The drawing under review shows one solid part. Ordinate dimensions are in mm from its lowest x, y, z. Give positions to 0.01 mm unless a question says otherwise; leave off trailing zeros. Write each loop counter-clockwise with the first axis right and the second up, starting at its lowest first coordinate (ties: lowest second). Pieces come first, ordered by that corner, then holes. Notation, with made-up numbers: (31.25, -2) -> (37.25, -2) arc R15 cw to (37.25, 11) -> close; hole circle Ø9 at (27, 40.5). An arc over 180 degrees is marked (long way). Write item = value, one per line.
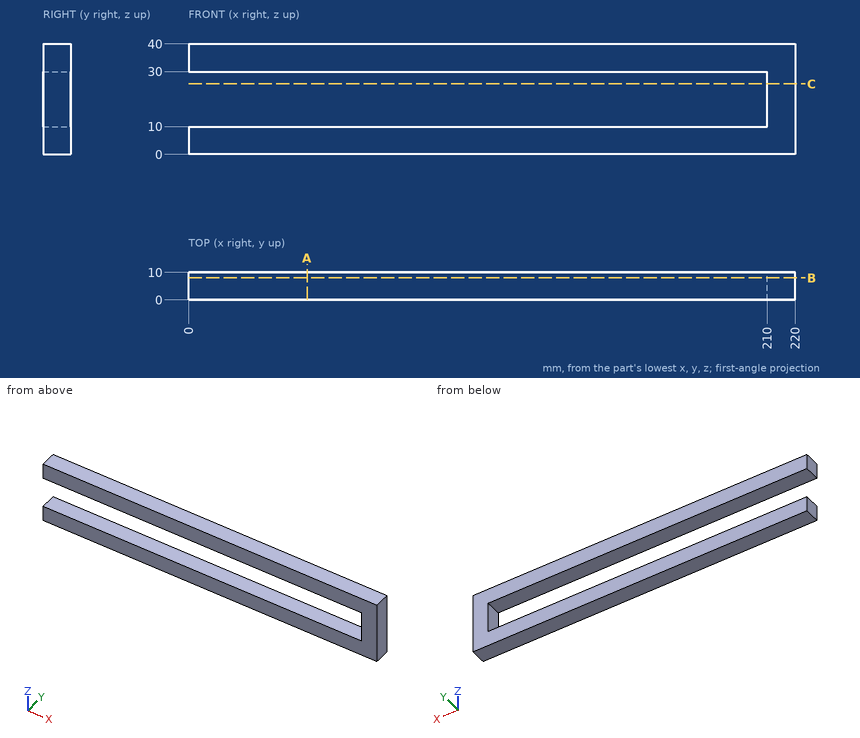
(1) Take a section at B-B (y = 8). Write out the cut boundary in (x, z).
Answers below:
outline = (0, 0) -> (220, 0) -> (220, 40) -> (0, 40) -> (0, 30) -> (210, 30) -> (210, 10) -> (0, 10) -> close
(2) For pin 1 (5 mm diameter, centred on x = 109, z = 29.5, fed in from +Y); pin 2 (10 mm diameter, centred on x = 51.5, z = 16.5, fed in from +Y), all flat-tipped, find the tip position at first contact; note any pin that passes through.
Answers below:
pin_1 = 10
pin_2 = through
(3) Take a section at C-C (z = 25.5). Write out the cut boundary in (x, y).
Answers below:
outline = (210, 0) -> (220, 0) -> (220, 10) -> (210, 10) -> close
(4) Take a section at A-A (x = 43). Write out the cut boundary in (y, z).
Answers below:
outline = (0, 0) -> (10, 0) -> (10, 10) -> (0, 10) -> close; (0, 30) -> (10, 30) -> (10, 40) -> (0, 40) -> close
(5) To check wall thickness, follow probe 1 along Z at (x, y) = (181, 8.75); probe 2 along X at (y, z) = (3.5, 11). State the ranges of each line that lie inside material, in increasing order.
Answers below:
probe_1 = 0 to 10, 30 to 40
probe_2 = 210 to 220
